Could you check a few things on this model? Use its own coordinates, in mm. A direction names the side the tool comes from. Give positions to 0.01 mm unless a question says otherwise; leave off trailing zeros. Loops run counter-clockwise (first coordinate to the right, second up) from the corner with the lowest first, then second, coordinate; pieces in that order, holes last. Notation, with made-up numbers: (35, -26.5) -> (71, -26.5) arc R20 cw to (71, -3.5) -> close; hole circle Ø2 at (-19, 80). An arc over 180 degrees is marked (long way). Write each question's results on one line, items separated by ' | '. Start each with the question number.
Q1. If we section it at C-C, the plane z = 1.6: List the corners of the cut face in (x, y) for me, plus the area to 3 significant figures.
Q2. Which directions (+Z, -Z, +X, -X, +Y, -Y) give clear straight access to the entire face, cutting with the end or side of a thin tool? Please do faces 4 (the face through (5, 21, 1)), 5 (the face through (-5, -21, 1)), 6 (the face through (5, -22, 1)).
Q3. If we section it at A-A, the plane x = 0: List the corners of the cut face in (y, z) for me, plus the area to 3 significant figures.
Q4. If we section it at B-B, the plane y = 0.5: List the corners of the cut face in (x, z) for me, plus the area to 3 significant figures.
Q5. We'd pull the mould along X, two halves only. Please class faces 1 (the face through (-0.59, 4.46, 1.48)), 2 (the face through (0, 23.5, 1)), 3 (the face through (6.137, 13.461, 1.479)): released by +X, released by -X, zero draft, split by the parting line, or undercut.
Q6. If we section it at D-D, the plane y = 20: List the corners of the cut face in (x, z) for me.
Q7. If I drill on line 1 along Y through (x, z) = (0, 0.85); line 2 along X through (y, z) = (-6.5, 0.65); line 3 along Y through (x, z) = (-6.25, 2.85), over which ranges is the centre line in solid material (lowest first)?
Q8. Will these pins go through, and if not, where does the flat tip stop? P1, Ø3.5, axis at x = -6.72, y = -6.72, coming from the +Z side; P2, Ø0.9, axis at y = 21, z = 1.5, coming from the +X side; P3, Ø3, axis at x = -5.66, y = 5.66, coming from the -Z side.
from build123d import *

# Parameters (mm, degrees)
F0_R     = 1.55
F0_R_2   = 1.6
F0_R_3   = 4.5
F1_DEPTH = 3


with BuildPart() as f1:
    # F0 (on Top) → F1 (new body)
    with BuildSketch(Plane.XY):
        with BuildLine():
            ThreePointArc((-5, 19.5), (-6.106463, 13.540947), (-9.278351, 8.376289))
            ThreePointArc((-9.278351, 8.376289), (-11.66682, 4.487238), (-12.5, 0))
            ThreePointArc((-12.5, 0), (-11.66682, -4.487238), (-9.278351, -8.376289))
            ThreePointArc((-9.278351, -8.376289), (-6.106463, -13.540947), (-5, -19.5))
            Line((-5, -19.5), (-5, -23.5))
            Line((-5, -23.5), (5, -23.5))
            Line((5, -23.5), (5, -19.5))
            ThreePointArc((5, -19.5), (6.106463, -13.540947), (9.278351, -8.376289))
            ThreePointArc((9.278351, -8.376289), (11.66682, -4.487238), (12.5, 0))
            ThreePointArc((12.5, 0), (11.66682, 4.487238), (9.278351, 8.376289))
            ThreePointArc((9.278351, 8.376289), (6.106463, 13.540947), (5, 19.5))
            Line((5, 19.5), (5, 23.5))
            Line((5, 23.5), (-5, 23.5))
            Line((-5, 23.5), (-5, 19.5))
        make_face()
        with Locations((-6.717514, -6.717514)):
            Circle(F0_R, mode=Mode.SUBTRACT)
        with Locations((0, -19.5)):
            Circle(F0_R_2, mode=Mode.SUBTRACT)
        with Locations((5.656854, -5.656854)):
            Circle(F0_R, mode=Mode.SUBTRACT)
        with Locations((-5.656854, 5.656854)):
            Circle(F0_R, mode=Mode.SUBTRACT)
        Circle(F0_R_3, mode=Mode.SUBTRACT)
        with Locations((6.717514, 6.717514)):
            Circle(F0_R, mode=Mode.SUBTRACT)
        with Locations((0, 19.5)):
            Circle(F0_R_2, mode=Mode.SUBTRACT)
    extrude(amount=F1_DEPTH)


solid = f1.part
Final values:
1) outline: (-12.5, 0) arc R12.5 ccw to (-9.28, -8.38) arc R16.6 cw to (-5, -19.5) -> (-5, -23.5) -> (5, -23.5) -> (5, -19.5) arc R16.6 cw to (9.28, -8.38) arc R12.5 ccw to (12.5, 0) arc R12.5 ccw to (9.28, 8.38) arc R16.6 cw to (5, 19.5) -> (5, 23.5) -> (-5, 23.5) -> (-5, 19.5) arc R16.6 cw to (-9.28, 8.38) arc R12.5 ccw to start; hole circle Ø3.1 at (-6.72, -6.72); hole circle Ø3.1 at (-5.66, 5.66); hole circle Ø9 at (0, 0); hole circle Ø3.2 at (0, -19.5); hole circle Ø3.2 at (0, 19.5); hole circle Ø3.1 at (5.66, -5.66); hole circle Ø3.1 at (6.72, 6.72) | area: 637 mm²
2) face 4: +Z, -Z, +X, +Y | face 5: +Z, -Z, -X, -Y | face 6: +Z, -Z, +X, -Y
3) outline: (-23.5, 0) -> (-21.1, 0) -> (-21.1, 3) -> (-23.5, 3) -> close; (-17.9, 0) -> (-4.5, 0) -> (-4.5, 3) -> (-17.9, 3) -> close; (4.5, 0) -> (17.9, 0) -> (17.9, 3) -> (4.5, 3) -> close; (21.1, 0) -> (23.5, 0) -> (23.5, 3) -> (21.1, 3) -> close | area: 94.8 mm²
4) outline: (-12.49, 0) -> (-4.47, 0) -> (-4.47, 3) -> (-12.49, 3) -> close; (4.47, 0) -> (12.49, 0) -> (12.49, 3) -> (4.47, 3) -> close | area: 48.1 mm²
5) face 1: undercut | face 2: zero draft | face 3: released by +X
6) outline: (-5, 0) -> (-1.52, 0) -> (-1.52, 3) -> (-5, 3) -> close; (1.52, 0) -> (5, 0) -> (5, 3) -> (1.52, 3) -> close
7) line 1: y = -23.5 to -21.1, -17.9 to -4.5, 4.5 to 17.9, 21.1 to 23.5 | line 2: x = -10.68 to -8.25, -5.18 to 4.36, 6.96 to 10.68 | line 3: y = -13.18 to -8.2, -5.24 to 4.22, 7.09 to 13.18
8) P1: stops at z = 3 | P2: stops at x = 5 | P3: passes through
